from build123d import *

# Parameters (mm, degrees)
SKETCH1_W            = 20
SKETCH1_H            = 26
SKETCH1_W_2          = 1.25
SKETCH1_H_2          = 15
BOSS_EXTRUDE5_DEPTH  = 5
SKETCH3_W            = 7
SKETCH3_H            = 26
BOSS_EXTRUDE6_DEPTH  = 40
CUT_EXTRUDE1_REACH   = 55.696
SKETCH5_R            = 11.2
SKETCH6_W            = 26
SKETCH6_H            = 5
BOSS_EXTRUDE8_DEPTH  = 14
SKETCH8_R            = 12
SKETCH8_R_2          = 7.5
BOSS_EXTRUDE9_DEPTH  = 2.5
SKETCH9_R            = 12
SKETCH9_R_2          = 7.5
BOSS_EXTRUDE10_DEPTH = 2.5
SKETCH7_W            = 12
SKETCH7_H            = 1.25
CUT_EXTRUDE2_DEPTH   = 10
BOSS_EXTRUDE11_DEPTH = 37.12
SKETCH14_R           = 2.25
SKETCH14_R_2         = 4.5
CUT_EXTRUDE4_DEPTH   = 10


with BuildPart() as part:
    # Sketch1 → Boss-Extrude5 (new body)
    with BuildSketch(Plane(origin=(0, 0, 0), x_dir=(1, 0, 0), z_dir=(0, 1, 0))):
        with Locations((10, 13)):
            Rectangle(SKETCH1_W, SKETCH1_H)
        with Locations((1.875, 13)):
            Rectangle(SKETCH1_W_2, SKETCH1_H_2, mode=Mode.SUBTRACT)
    boss_extrude5 = extrude(amount=BOSS_EXTRUDE5_DEPTH)

    # Sketch3 → Boss-Extrude6 (add)
    with BuildSketch(Plane(origin=(0, 5, 0), x_dir=(1, 0, 0), z_dir=(0, 1, 0))):
        with Locations((10, 13)):
            Rectangle(SKETCH3_W, SKETCH3_H)
    boss_extrude6 = extrude(amount=BOSS_EXTRUDE6_DEPTH)

    # Sketch5 → Cut-Extrude1 (cut, up to next)
    with BuildSketch(Plane(origin=(13.5, 0, 0), x_dir=(0, 0, -1), z_dir=(1, 0, 0)), mode=Mode.PRIVATE) as cut_extrude1_sk1:
        with Locations((13, 20)):
            Circle(SKETCH5_R)
    cut_extrude1_tool1 = extrude(cut_extrude1_sk1.sketch, amount=-CUT_EXTRUDE1_REACH, mode=Mode.PRIVATE) & part.part
    # Sketch5 → Cut-Extrude1 (cut, up to next)
    with BuildSketch(Plane(origin=(13.5, 0, 0), x_dir=(0, 0, -1), z_dir=(1, 0, 0)), mode=Mode.PRIVATE) as cut_extrude1_sk2:
        with BuildLine():
            Line((0, 27.483314774), (0, 45))
            Line((0, 45), (26, 45))
            Line((26, 45), (26, 27.483314774))
            ThreePointArc((26, 27.483314774), (13, 35), (0, 27.483314774))
        make_face()
    cut_extrude1_tool2 = extrude(cut_extrude1_sk2.sketch, amount=-CUT_EXTRUDE1_REACH, mode=Mode.PRIVATE) & part.part
    cut_extrude1_1 = cut_extrude1_tool1.solids().sort_by_distance((13.5, 20, -13))[0]
    add(cut_extrude1_1, mode=Mode.SUBTRACT)
    cut_extrude1_2 = cut_extrude1_tool2.solids().sort_by_distance((13.5, 38.725293, -13))[0]
    add(cut_extrude1_2, mode=Mode.SUBTRACT)
    cut_extrude1 = cut_extrude1_1 + cut_extrude1_2  # Cut-Extrude1 as one shape, for the pattern or mirror that repeats it

    # Sketch6 → Boss-Extrude8 (add)
    with BuildSketch(Plane(origin=(20, 0, 0), x_dir=(0, 0, -1), z_dir=(1, 0, 0))):
        with Locations((13, 2.5)):
            Rectangle(SKETCH6_W, SKETCH6_H)
    boss_extrude8 = extrude(amount=BOSS_EXTRUDE8_DEPTH)

    # Mirror5: Boss-Extrude5, Boss-Extrude6, Cut-Extrude1, Boss-Extrude8 across plane
    add(boss_extrude5.mirror(Plane.ZY.offset(-34)))
    add(boss_extrude6.mirror(Plane.ZY.offset(-34)))
    add(cut_extrude1.mirror(Plane.ZY.offset(-34)), mode=Mode.SUBTRACT)
    add(boss_extrude8.mirror(Plane.ZY.offset(-34)))

    # Sketch8 → Boss-Extrude9 (add)
    with BuildSketch(Plane.ZY.offset(-6.5)):
        with Locations(Location((-13, 20, 0), (0, 0, 180))):
            Circle(SKETCH8_R)
        with Locations((-13, 20)):
            Circle(SKETCH8_R_2, mode=Mode.SUBTRACT)
    extrude(amount=BOSS_EXTRUDE9_DEPTH)

    # Sketch9 → Boss-Extrude10 (add)
    with BuildSketch(Plane.ZY.offset(-54.5)):
        with Locations(Location((-13, 20, 0), (0, 0, 180))):
            Circle(SKETCH9_R)
        with Locations((-13, 20)):
            Circle(SKETCH9_R_2, mode=Mode.SUBTRACT)
    extrude(amount=BOSS_EXTRUDE10_DEPTH)

    # Sketch7 → Cut-Extrude2 (cut)
    with BuildSketch(Plane(origin=(0, 5, 0), x_dir=(1, 0, 0), z_dir=(0, 1, 0))):
        with Locations((22, 1.875)):
            Rectangle(SKETCH7_W, SKETCH7_H)
        with Locations((46, 1.875)):
            Rectangle(SKETCH7_W, SKETCH7_H)
        with Locations((46, 24.125)):
            Rectangle(SKETCH7_W, SKETCH7_H)
        with Locations((22, 24.125)):
            Rectangle(SKETCH7_W, SKETCH7_H)
    extrude(amount=-CUT_EXTRUDE2_DEPTH, mode=Mode.SUBTRACT)

    # Sketch10 → Boss-Extrude11 (add)
    with BuildSketch(Plane.XY):
        Polygon((51, 0), (68, 0), (68, 5), (61.5, 5), (61.5, 47.8), (57.5, 47.8), (57.5, 5), (51, 5), align=None)
    extrude(amount=BOSS_EXTRUDE11_DEPTH)

    # Sketch14 → Cut-Extrude4 (cut)
    with BuildSketch(Plane(origin=(61.5, 0, 0), x_dir=(0, 0, -1), z_dir=(1, 0, 0))):
        Polygon((-37.12, 51.83243557), (-37.12, 47.8), (-18.56, 47.8), (0, 47.8), (0, 51.83243557), align=None)
        with BuildLine():
            Line((0, 47.8), (-18.56, 47.8))
            ThreePointArc((-18.56, 47.8), (-8.484558377, 45.75747818), (0, 39.952421039))
            Line((0, 39.952421039), (0, 47.8))
        make_face()
        with BuildLine():
            Line((-37.12, 47.8), (-37.12, 39.952421039))
            ThreePointArc((-37.12, 39.952421039), (-28.635441623, 45.75747818), (-18.56, 47.8))
            Line((-18.56, 47.8), (-37.12, 47.8))
        make_face()
        with Locations((-18.556883399, 43.896979327)):
            Circle(SKETCH14_R)
        with Locations((-10.556883399, 26.396979327)):
            Circle(SKETCH14_R_2)
        with Locations((-18.556883399, 8.896979327)):
            Circle(SKETCH14_R)
    extrude(amount=-CUT_EXTRUDE4_DEPTH, mode=Mode.SUBTRACT)


solid = part.part
The listing builds one solid part. Answer for the finished solid, in the listing's coordinates (mm). A direction names the side the tool comes from. Give positions to 0.01 mm unless a question says otherwise; leave off trailing zeros. Loops run counter-clockwise (first coordinate to the right, second up) from the corner with the lowest first, then second, coordinate; pieces in that order, holes last. Notation, with made-up numbers: (62, -7.75) - (93, -7.75) arc R8 ccw to (93, -2.75) - close; hole circle Ø8 at (72.25, 76). An arc over 180 degrees is marked (long way). Answer as a JSON object with one key per item and string values.
1. A cutting plane is placed at D-D (x = 37). Write down the section's boundary in (y, z), then the cut area to 3 significant figures.
Determined:
{"outline": "(0, -26) - (5, -26) - (5, 0) - (0, 0) - close", "area": "130 mm²"}
2. A cutting plane is placed at A-A (y = 20). Give the number of separate pieces and of enclosed holes in the cut face, then the cut area to 3 significant figures.
Determined:
{"separate pieces": "4", "enclosed holes": "0", "area": "244 mm²"}
3. For a pull along Z with two mould halves and no side action, classify faces 5 (the flat face through (36, 5, -9)), 6 (the cylindrical face through (59.53, 23.66, 14.13)), 7 (the flat face through (18.1, 4.5, 0)), 8 (the flat face through (46, 3, -24.75)) as pulls with the +Z half, pulls with the -Z half, needs draft (parallel to the pull), parting line crosses it, or undercut.
Determined:
{"face 5": "needs draft", "face 6": "undercut", "face 7": "pulls with the +Z half", "face 8": "undercut"}
4. Find the intervals of material crossed by L1, parallel to Z at x = 20, y = 3.5; L2, parallel to X at y = 30.5, z = -20.5; L3, parallel to X at y = 26, z = 34.5, in increasing order. Write a range as [from, to].
Determined:
{"L1": "[-26, -24.75], [-23.5, -2.5], [-1.25, 0]", "L2": "[6.5, 13.5], [54.5, 61.5]", "L3": "[57.5, 61.5]"}
5. Flat-ended cylindrical pins translate along their axes: pin 1 Ø2 at (x, z) = (65.5, 9.5) entering from +Y; pin 2 Ø3 at (y, z) = (34, 12.5) entering from -X; pin 3 Ø14.5 at (y, z) = (26.4, 10.56) entering from +X. Find the tip coordinate at first contact, or state that the pin passes through.
Determined:
{"pin 1": "y = 5", "pin 2": "x = 57.5", "pin 3": "x = 61.5"}
6. For faces 1 (the flat face through (6.5, 8.8, -17.8)), 2 (the cylindrical face through (57.951, 10.064, -18.168)), 3 (the flat face through (22, 3, -1.25)), 4 (the flat face through (59, 34, 0)), determine the directions among +Z, -Z, +X, -X, +Y, -Y from which every point of the face is accessible in a straight line to the end or side of a thin tool.
Determined:
{"face 1": "-X", "face 2": "+X", "face 3": "+Y, -Y", "face 4": "+X, -X, +Y"}
